The listing builds one solid part. Answer for the finished solid, in the listing's coordinates (mm). Face numbers are marked on the shaded views. A direction names the side the tool comes from. Coordinates: 2 decimals unless noted, no trailing zeros. Write each loop counter-clockwise with the first axis right and the second up, starting at its lowest first coordinate (ties: lowest second). Pieces come first, ordered by that corner, then holes. Notation, with made-up numbers: M 15.5,-40 L 25.5,-40 A22 ccw 25.5,-26 Z; hole C 49.5,-3.75 d8. An arc over 180 degrees is marked long. Answer as a JSON object with one key per item and string values. Group by question number.
from build123d import *

# Parameters (mm, degrees)
SKETCH2_W           = 12.95
SKETCH2_H           = 6.35
BOSS_EXTRUDE1_DEPTH = 2.54
SKETCH3_W           = 5.21
SKETCH3_H           = 6.35
SKETCH3_W_2         = 4.56
BOSS_EXTRUDE2_DEPTH = 8
SKETCH5_R           = 0.26
BOSS_EXTRUDE5_DEPTH = 2.5
SKETCH6_W           = 8.4
SKETCH6_H           = 6.35
BOSS_EXTRUDE6_DEPTH = 2.03


with BuildPart() as part:
    # Sketch2 → Boss-Extrude1 (new body)
    with BuildSketch(Plane(origin=(0, 0, 0), x_dir=(1, 0, 0), z_dir=(0, 1, 0))):
        Rectangle(SKETCH2_W, SKETCH2_H)
    extrude(amount=BOSS_EXTRUDE1_DEPTH)

    # Sketch3 → Boss-Extrude2 (add)
    with BuildSketch(Plane(origin=(0, 2.54, 0), x_dir=(1, 0, 0), z_dir=(0, 1, 0))):
        with Locations((-3.87, 0)):
            Rectangle(SKETCH3_W, SKETCH3_H)
        with Locations((4.195, 0)):
            Rectangle(SKETCH3_W_2, SKETCH3_H)
    extrude(amount=BOSS_EXTRUDE2_DEPTH)

    # Sketch5 → Boss-Extrude5 (add)
    with BuildSketch(Plane.XZ):
        with Locations((-3.74, -1.27)):
            Circle(SKETCH5_R)
        with Locations((-3.74, 1.27)):
            Circle(SKETCH5_R)
        with Locations((4.39, -1.27)):
            Circle(SKETCH5_R)
        with Locations((4.39, 1.27)):
            Circle(SKETCH5_R)
    extrude(amount=BOSS_EXTRUDE5_DEPTH)

    # Sketch6 → Boss-Extrude6 (add)
    with BuildSketch(Plane.ZY.offset(6.475)):
        with Locations((-7.375, 5.965)):
            Rectangle(SKETCH6_W, SKETCH6_H)
        with BuildLine():
            ThreePointArc((-8.436140087, 4.375), (-10.026140087, 5.965), (-8.436140087, 7.555))
            Line((-8.436140087, 7.555), (-5.776140087, 7.555))
            ThreePointArc((-5.776140087, 7.555), (-4.651840305, 7.089299782), (-4.186140087, 5.965))
            ThreePointArc((-4.186140087, 5.965), (-4.651840305, 4.840700218), (-5.776140087, 4.375))
            Line((-5.776140087, 4.375), (-8.436140087, 4.375))
        make_face(mode=Mode.SUBTRACT)
        with Locations((7.375, 5.965)):
            Rectangle(SKETCH6_W, SKETCH6_H)
        with BuildLine():
            ThreePointArc((5.78, 4.375), (4.19, 5.965), (5.78, 7.555))
            Line((5.78, 7.555), (8.44, 7.555))
            ThreePointArc((8.44, 7.555), (9.564299782, 7.089299782), (10.03, 5.965))
            ThreePointArc((10.03, 5.965), (9.564299782, 4.840700218), (8.44, 4.375))
            Line((8.44, 4.375), (5.78, 4.375))
        make_face(mode=Mode.SUBTRACT)
    extrude(amount=-BOSS_EXTRUDE6_DEPTH)


solid = part.part
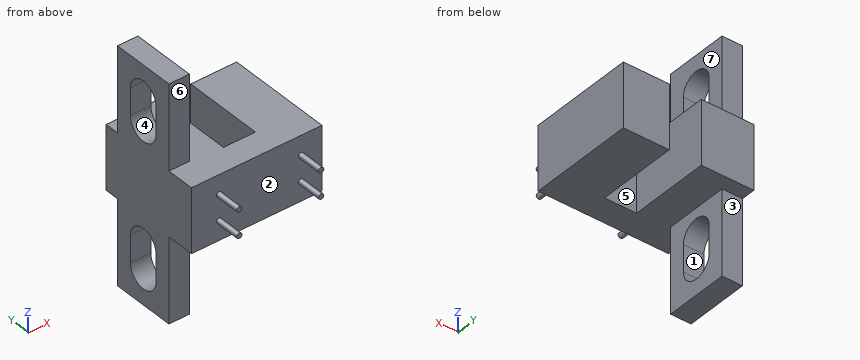
Item 1: A cutting plane is placed at B-B, the plane y = 3.5. Write down the section's boundary in (x, z) (3 decimals), and give its area (3 significant figures).
Item 2: Flat-ended cylindrical pins translate along their axes: pin 1 Ø7 at (y, z) = (6.5, -7) entering from +X (3 decimals); pin 2 Ø1 at (x, z) = (-6, -6.5) entering from +Y; pin 3 Ø1.6 at (x, z) = (-5.5, -6) entering from -Y; pin 4 Ø5.5 at (x, y) = (-3, 7.5) entering from -Z (3 decimals). Find the tip coordinate at first contact, or state that the pin passes through.
Item 3: For a pull along Y with two mould halves and no side action, classify the marked faces 1, 2 and 3 as +Y half, -Y half, draft (parallel to the pull), parting line (faces both ways), or undercut.
Item 4: A tool of negligible diameter and unlimited length cuts with its end or side. For the marked faces 4, 5, 6 and 7, from which of +Z, -Z, +X, -X, +Y, -Y can it reach the whole face along a straight path? Write none if from no direction.
Item 5: A cutting plane is placed at C-C, the plane y = 5.5. Write down the section's boundary in (x, z) (3 decimals).
Item 6: A cutting plane is placed at A-A, the plane z = 7.5. Write down the section's boundary in (x, y) (3 decimals).
Item 7: A cutting plane is placed at D-D, the plane x = -3.74. Write down the section's boundary in (y, z) (3 decimals), and give its area (3 significant figures).
Item 8: Consider L1, parallel to Z at x = -5.25, y = 0.5 (3 decimals); L2, parallel to X at y = 7.75, z = 6.25 (3 decimals); L3, parallel to Y at x = 4.25, z = -0.75. Determine where each line is inside the solid, lowest interval first. Write a range as from..to.
Answer:
{
 "1": {"outline": "M -6.475,-11.575 L -4.445,-11.575 L -4.445,-3.175 L -1.265,-3.175 L -1.265,3.175 L -4.445,3.175 L -4.445,11.575 L -6.475,11.575 Z; M 1.915,-3.175 L 6.475,-3.175 L 6.475,3.175 L 1.915,3.175 Z", "area": "96.1 mm2"},
 "2": {"pin 1": "x = -4.445", "pin 2": "y = 9.14", "pin 3": "y = 2.79", "pin 4": "z = -11.575"},
 "3": {"face 1": "undercut", "face 2": "-Y half", "face 3": "+Y half"},
 "4": {"face 4": "+X, -X", "face 5": "+Z, -Z, +Y", "face 6": "+Z, +X, -X, -Y", "face 7": "+Z, +X, +Y, -Y"},
 "5": {"outline": "M -6.475,-11.575 L -4.445,-11.575 L -4.445,-9.957 L -6.475,-9.957 Z; M -6.475,-4.256 L -4.445,-4.256 L -4.445,-3.175 L -1.265,-3.175 L -1.265,3.175 L -4.445,3.175 L -4.445,4.26 L -6.475,4.26 Z; M -6.475,9.96 L -4.445,9.96 L -4.445,11.575 L -6.475,11.575 Z; M 1.915,-3.175 L 6.475,-3.175 L 6.475,3.175 L 1.915,3.175 Z"},
 "6": {"outline": "M -6.475,2.79 L -4.445,2.79 L -4.445,4.375 L -6.475,4.375 Z; M -6.475,7.555 L -4.445,7.555 L -4.445,9.14 L -6.475,9.14 Z"},
 "7": {"outline": "M -2.5,-1.53 L 0,-1.53 L 0,-3.175 L 10.54,-3.175 L 10.54,3.175 L 0,3.175 L 0,1.53 L -2.5,1.53 L -2.5,1.01 L 0,1.01 L 0,-1.01 L -2.5,-1.01 Z", "area": "69.5 mm2"},
 "8": {"L1": "-3.175..3.175", "L2": "-6.475..-4.445", "L3": "0..10.54"}
}
